Model file for the job. Use its own axes, mm. A direction names the side the tool comes from. Round coordinates to 2 decimals unless told otherwise and drop trailing zeros. Loops run counter-clockwise (first coordinate to the right, second up) from the corner with the lowest first, then second, coordinate; pieces in that order, holes last. Notation, with made-up numbers: M 5,7.5 L 16,7.5 A19 ccw 16,17.5 Z; hole C 14,-3 d6. An arc over 180 degrees is marked long. Use a Markdown table: item, result. Add a question column.
Item 1: Wall check: L1, parallel to Y at x = 21, z = 0; L2, parallel to Y at x = 124, z = 0; L3, parallel to X at y = 4, z = 7. Give the ranges that are in metal, low to high. Write a range as from..to.
Item 2: Saw through at A-A on x = 305.5. Write the cut outline in (y, z), then the cut area to 3 significant figures.
Item 3: Tool access for faces 4 (the cylindrical face through (22.22, 13.18, -2.93)), 5 (the flat face through (425, 0, 8.5)), 6 (the flat face through (425, 0, -8.5)): list every direction of +Z, -Z, +X, -X, +Y, -Y with a clear straight run to the whole face (end or side of a thin tool).
Item 4: Pin check, flat tips, straight feed: P1, Ø6, axis at y = 4.5, z = -2, coming from the -X side; P2, Ø4, axis at x = 88, z = 0, coming from the -Y side; P3, Ø6, axis at y = 15, z = 0.5, coming from the +X side; P4, Ø3, axis at x = 119.5, y = -17.5, coming from the -Z side. Stop position of each tip, or through.
Item 5: Two-plate mould, pull along Y, no slides. Class faces 1 (the flat face through (100, 0, -11)), 2 (the flat face through (128.5, 10, -3)), 3 (the cylindrical face through (284, 0, 10)): +Y half, -Y half, draft (parallel to the pull), parting line (faces both ways), or undercut.
Autodesk Inventor part; units mm, degrees
ref_plane "Płaszczyzna konstrukcyjna1" through (43, 0, 0) normal (-1, 0, 0) x (0, 0, 1)
ref_plane "Płaszczyzna konstrukcyjna2" through (10, 0, 0) normal (-1, 0, 0) x (0, 0, 1)
ref_plane "Płaszczyzna konstrukcyjna3" through (115.5, 0, 0) normal (1, 0, 0) x (0, 0, -1)
sketch "Szkic1" plane through (0, 0, 0) normal (1, 0, 0) x (0, 1, 0)
  circle A0 centre (0, 0) radius 7
  dimension "d0" = 14
extrude "Wyciągnięcie proste1" add sketch "Szkic1" along normal blind 100
sketch "Szkic2" plane through (100, 0, 0) normal (1, 0, 0) x (0, 0, -1)
  circle A0 centre (0, 0) radius 25.5
  dimension "d3" = 51
extrude "Wyciągnięcie proste2" add sketch "Szkic2" against normal blind 3
ref_plane "Płaszczyzna konstrukcyjna1" through (43, 0, 0) normal (-1, 0, 0) x (0, 0, 1)
sketch "Szkic3" plane through (43, 0, 0) normal (-1, 0, 0) x (0, 0, 1)
  circle A0 centre (0, 0) radius 25.5
extrude "Wyciągnięcie proste3" add sketch "Szkic3" along normal blind 3
sketch "Szkic4" plane through (40, 0, 0) normal (-1, 0, 0) x (0, 0, 1)
  circle A0 centre (0, 0) radius 10
  dimension "d9" = 20
extrude "Wyciągnięcie proste4" add sketch "Szkic4" along normal blind 9
sketch "Szkic5" plane through (31, 0, 0) normal (-1, 0, 0) x (0, 0, 1)
  circle A0 centre (0, 0) radius 13.5
  dimension "d12" = 27
extrude "Wyciągnięcie proste5" add sketch "Szkic5" along normal blind 11
fillet "Zaokrąglenie1" radius 8 1 edges at (31, 0, -13.5)
ref_plane "Płaszczyzna konstrukcyjna2" through (10, 0, 0) normal (-1, 0, 0) x (0, 0, 1)
sketch "Szkic6" plane through (10, 0, 0) normal (-1, 0, 0) x (0, 0, 1)
  circle A0 centre (0, 0) radius 14.5
  dimension "d19" = 29
extrude "Wyciągnięcie proste6" add sketch "Szkic6" against normal blind 1
sketch "Szkic7" plane through (11, 0, 0) normal (1, 0, 0) x (0, 0, -1)
  circle A0 centre (0, 0) radius 15
  dimension "d22" = 30
extrude "Wyciągnięcie proste7" add sketch "Szkic7" along normal blind 1
sketch "Szkic8" plane through (12, 0, 0) normal (1, 0, 0) x (0, 0, -1)
  circle A0 centre (0, 0) radius 7
  circle A1 centre (0, 0) radius 15.75
  circle A2 centre (0, 0) radius 13.5
  circle A3 centre (0, 0) radius 14.5
  dimension "d25" = 31.5
extrude "Wyciągnięcie proste8" add sketch "Szkic8" along normal blind 13 contours A1
extrude "Wyciągnięcie proste9" add sketch "Szkic8" along normal blind 7.75 contours A0 | A2 | A3
sketch "Szkic9" plane through (100, 0, 0) normal (1, 0, 0) x (0, 0, -1)
  circle A0 centre (0, 0) radius 7
  circle A1 centre (0, 0) radius 10
  dimension "d30" = 14
  dimension "d33" = 20
extrude "Wyciągnięcie proste10" add sketch "Szkic9" along normal blind 23 contours A0
extrude "Wyciągnięcie proste11" add sketch "Szkic9" along normal blind 9
sketch "Szkic10" plane through (109, 0, 0) normal (1, 0, 0) x (0, 0, -1)
  circle A0 centre (0, 0) radius 25.5
  circle A1 centre (0, 0) radius 13.5
  dimension "d36" = 27
extrude "Wyciągnięcie proste12" add sketch "Szkic10" along normal blind 11 contours A1
fillet "Zaokrąglenie2" radius 8 1 edges at (109, 0, 13.5)
ref_plane "Płaszczyzna konstrukcyjna3" through (115.5, 0, 0) normal (1, 0, 0) x (0, 0, -1)
sketch "Szkic11" plane through (115.5, 0, 0) normal (1, 0, 0) x (0, 0, -1)
  circle A0 centre (0, 0) radius 15.75
  circle A1 centre (0, 0) radius 14.5
  dimension "d41" = 31.5
  dimension "d42" = 29
extrude "Wyciągnięcie proste13" add sketch "Szkic11" along normal blind 13
sketch "Szkic12" plane through (123, 0, 0) normal (1, 0, 0) x (0, 0, -1)
  circle A0 centre (0, 0) radius 10
  dimension "d45" = 20
extrude "Wyciągnięcie proste14" add sketch "Szkic12" along normal blind 350
ref_plane "Płaszczyzna konstrukcyjna4" through (128.5, 0, 0) normal (1, 0, 0) x (0, 0, -1)
sketch "Szkic13" plane through (128.5, 0, 0) normal (1, 0, 0) x (0, 0, -1)
  circle A0 centre (0, 0) radius 15.75
extrude "Wyciągnięcie proste15" add sketch "Szkic13" along normal blind 8
fillet "Zaokrąglenie3" radius 8 1 edges at (136.5, 0, 15.75)
sketch "Szkic14" plane through (473, 0, 0) normal (1, 0, 0) x (0, 0, -1)
  circle A0 centre (0, 0) radius 7.5
  circle A1 centre (0, 0) radius 18.8953
  dimension "d52" = 15
extrude "Wyciągnięcie proste16" cut sketch "Szkic14" against normal blind 35
thread "Gwint2"
chamfer "Faza1" distance 2 angle 45 2 edges at (473, 0, 7.5) (438, 0, 10)
ref_plane "Płaszczyzna konstrukcyjna5" through (123, 10, 0) normal (0, 1, 0) x (-1, 0, 0)
sketch "Szkic15" plane through (123, 10, 0) normal (0, 1, 0) x (-1, 0, 0)
  line L0 (-290.266, 8.5) -> (-315.266, 8.5)
  line L1 (-315.266, 8.5) -> (-315.266, -8.5)
  line L2 (-315.266, -8.5) -> (-290.266, -8.5)
  line L3 (-290.266, -8.5) -> (-290.266, 8.5)
  line L4 (-290.266, 8.5) -> (-315.266, -8.5) construction
  line L5 (-315.266, 8.5) -> (-290.266, -8.5) construction
  line L6 (-317.1784, 11.3555) -> (-288.3535, 11.3555)
  line L7 (-288.3535, 11.3555) -> (-288.3535, -11.3555)
  line L8 (-288.3535, -11.3555) -> (-317.1784, -11.3555)
  line L9 (-317.1784, -11.3555) -> (-317.1784, 11.3555)
  line L10 (-317.1784, 11.3555) -> (-288.3535, -11.3555) construction
  line L11 (-288.3535, 11.3555) -> (-317.1784, -11.3555) construction
  line L12 (-290.266, -8.5) -> (-288.3535, -11.3555)
  line L13 (-290.266, 8.5) -> (-288.3535, 11.3555)
  line L14 (-315.266, -8.5) -> (-317.1784, -8.5)
  line L15 (-315.266, 8.5) -> (-317.1784, 8.5)
  point P0 (123, 0)
  point P1 (-302.766, 0)
  dimension "d60" = 25
  dimension "d61" = 17
extrude "Wyciągnięcie proste17" cut sketch "Szkic15" against normal blind 35 contours L0 L15 L9 L6 L13 | L12 L8 L9 L14 L2
thread "Gwint4"
chamfer "Faza3" distance 2 angle 45 1 edges at (0, -7, 0)
properties part number "tłoczysko"
Entries:
| question | item | result |
|---|---|---|
| 1 | L1 | -15.75..-14.5, -13.5..13.5, 14.5..15.75 |
| 1 | L2 | -15.75..-14.5, -10..10, 14.5..15.75 |
| 1 | L3 | 10..19.75, 20..43, 97..120, 123..437.94 |
| 2 | outline | C 0,0 d20 |
| 2 | area | 314 mm2 |
| 3 | face 4 | none |
| 3 | face 5 | +Z, +X, +Y, -Y |
| 3 | face 6 | -Z, +X, +Y, -Y |
| 4 | P1 | x = 0 |
| 4 | P2 | y = -7 |
| 4 | P3 | x = 135.6 |
| 4 | P4 | through |
| 5 | face 1 | draft |
| 5 | face 2 | undercut |
| 5 | face 3 | parting line |
